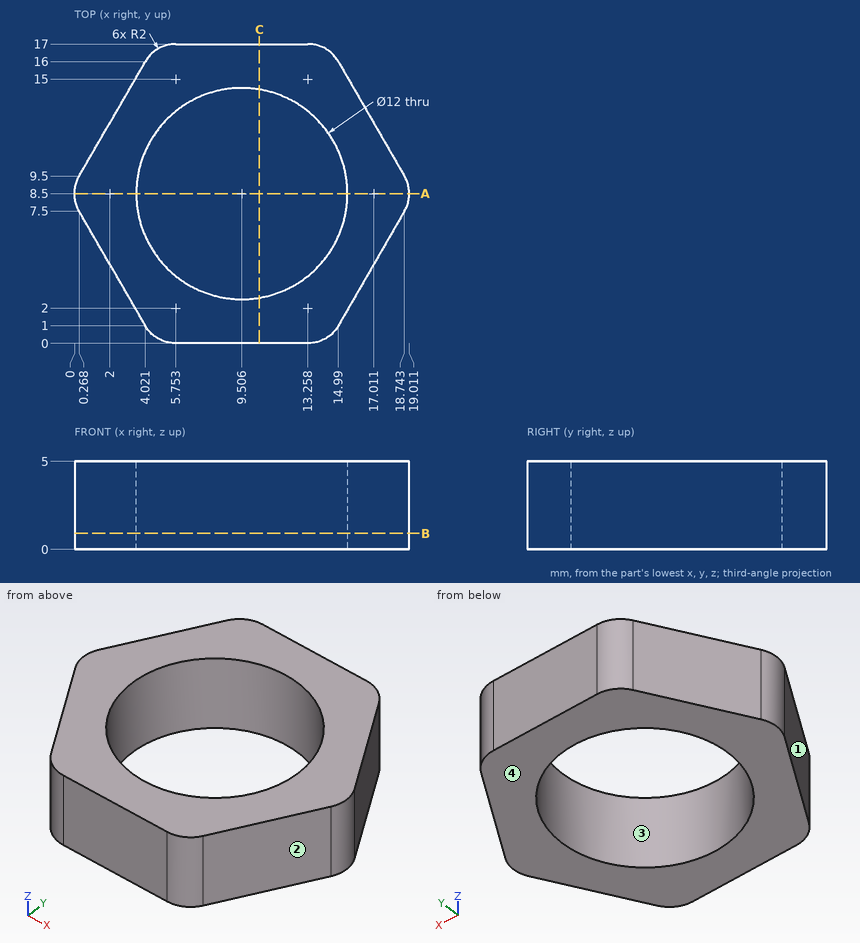
Design review of the part shown in the three views and the two pictorial views. Dimensions are in mm from the part's minimum x, y and z. Round coordinates to 2 decimals unless told otherwise and drop trailing zeros. Write each loop counter-clockwise with the first axis right and the second up, starting at its lowest first coordinate (ties: lowest second). Pieces come first, ordered by that corner, then holes. Notation, with made-up numbers: M -17,43.5 L 11,43.5 A24 ccw 11,79.5 Z; hole C 7.5,-30 d7. An arc over 180 degrees is marked long. One line per item, written item: value. Start each with the question number.
1. Take a section at A-A on y = 8.5. State the section outline as (x, z) points (1 decimal).
2. To check wall thickness, follow probe 1 along Y at (x, z) = (9.75, 2.55) (1 decimal); probe 2 along Y at (x, z) = (11, 3.25); probe 3 along X at (y, z) = (13.75, 4.85) (1 decimal). State the ranges of each line that lie inside material, in increasing order. Write a range as from..to.
3. Take a section at B-B on z = 0.9. State the section outline as (x, y) points (1 decimal).
4. Clearance check with flat-ended pins moving along their axes: P1, Ø7, axis at x = 9.51, y = 8.5, coming from the -Z side; P2, Ø3, axis at y = 9.5, z = 3.5, coming from the -X side; P3, Ø1.5, axis at y = 6, z = 3.5, coming from the +X side. State where each tip first meets the part, or that it passes through.
5. Take a section at C-C on x = 10.5. State the section outline as (y, z) points.
6. Draft analysis for pull direction X (two halves, no side actions). For the marked faces 1, 2, 3 and 4, state which applies: pulls with the +X half, pulls with the -X half, needs draft (parallel to the pull), parting line crosses it, or undercut.
Computed:
1. outline: M 0,0 L 3.5,0 L 3.5,5 L 0,5 Z; M 15.5,0 L 19,0 L 19,5 L 15.5,5 Z
2. probe 1: y = 0..2.5, 14.5..17
2. probe 2: y = 0..2.69, 14.31..17
2. probe 3: x = 2.7..6.6, 12.4..16.3
3. outline: M 0.3,7.5 L 4,1 A2 ccw 5.8,0 L 13.3,0 A2 ccw 15,1 L 18.7,7.5 A2 ccw 18.7,9.5 L 15,16 A2 ccw 13.3,17 L 5.8,17 A2 ccw 4,16 L 0.3,9.5 A2 ccw Z; hole C 9.5,8.5 d12
4. P1: passes through
4. P2: stops at x = 0
4. P3: stops at x = 18.31
5. outline: M 0,0 L 2.58,0 L 2.58,5 L 0,5 Z; M 14.42,0 L 17,0 L 17,5 L 14.42,5 Z
6. face 1: pulls with the -X half
6. face 2: pulls with the +X half
6. face 3: undercut
6. face 4: needs draft
